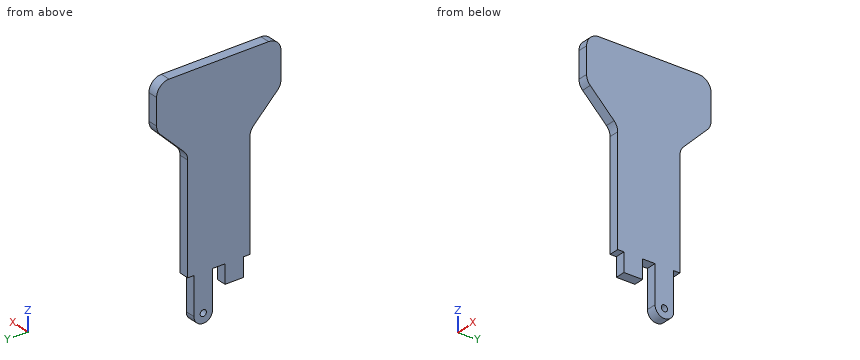
Autodesk Inventor part; units mm, degrees
ref_plane "YZ Plane" through (0, 0, 0) normal (1, 0, 0) x (0, 1, 0)
ref_plane "XZ Plane" through (0, 0, 0) normal (0, 1, 0) x (-1, 0, 0)
ref_plane "XY Plane" through (0, 0, 0) normal (0, 0, 1) x (1, 0, 0)
sketch "Sketch1" plane through (0, 0, 0) normal (1, 0, 0) x (0, 1, 0)
  line L0 (0, 0) -> (1, 0)
  line L1 (1, 0) -> (1, -3)
  line L2 (1, -3) -> (4, -3)
  line L3 (4, -3) -> (4, 0)
  line L4 (4, 0) -> (5, 0)
  line L5 (5, 0) -> (5, 18)
  line L6 (5, 18) -> (10, 23)
  line L7 (10, 23) -> (10, 30)
  line L8 (10, 30) -> (0, 30)
  line L9 (0, 30) -> (0, 0)
  dimension "d0" = 1
  dimension "d1" = 3
  dimension "d2" = 1
  dimension "d3" = 3
  dimension "d4" = 30
  dimension "d5" = 7
  dimension "d6" = 45
  dimension "d7" = 10
extrude "Extrusion1" add sketch "Sketch1" along normal blind 1.6
mirror "Mirror1" about plane through (0, 0, 30) normal (0, -1, 0) of "Extrusion1"
fillet "Fillet1" radius 2 6 edges at (0.8, 10, 30) (0.8, 10, 23) (0.8, -10, 30) (0.8, -10, 23) (0.8, -5, 18) (0.8, 5, 18)
sketch "Sketch2" plane through (1.6, 0, 0) normal (1, 0, 0) x (0, 0, -1)
  line L0 (0, 1) -> (3, 1)
  line L1 (3, 1) -> (3, 4)
  arc A0 (6, 1) -> (6, 4) centre (6, 2.5) ccw
  line L2 (3, 4) -> (6, 4)
  line L3 (3, 1) -> (6, 1)
  circle A1 centre (6, 2.5) radius 0.5
  point P0 (0, 0)
  dimension "d11" = 3
  dimension "d12" = 3
  dimension "d13" = 1
extrude "Extrusion2" add sketch "Sketch2" against normal up to surface (1.6 mm away)
sketch "Sketch3" plane through (1.6, 0, 0) normal (1, 0, 0) x (0, 0, -1)
  line L0 (-30, 10) -> (7.5, 10) construction
  line L1 (7.5, 10) -> (7.5, -9.9928) construction
  line L2 (7.5, -9.9928) -> (-30, -9.9928) construction
  line L3 (-30, -9.9928) -> (-30, 10) construction
  line L4 (-23.8284, 10) -> (-28, 10)
  line L5 (-30, 8) -> (-30, -8)
  arc A0 (6, 1) -> (6, 4) centre (6, 2.5) ccw
  point P0 (0, 0)
  dimension "d17" = 1.5
  dimension "d18" = 1.5
decal "Decal1"
sketch "Sketch4" plane through (0, 0, 0) normal (-1, 0, 0) x (0, 0, 1)
  line L0 (-7.5, 10) -> (30, 10) construction
  line L1 (30, 10) -> (30, -9.9928) construction
  line L2 (30, -9.9928) -> (-7.5, -9.9928) construction
  line L3 (-7.5, -9.9928) -> (-7.5, 10) construction
  line L4 (30, 8) -> (30, -8)
  line L5 (23.8284, 10) -> (28, 10)
  arc A0 (-6, 4) -> (-6, 1) centre (-6, 2.5) ccw
  point P0 (0, 0)
  dimension "d20" = 1.5
decal "Decal2"
equation "\"d17\" = d18"
equation "\"d20\" = d18"
properties part number "KeyerPaddle"
Geometry check sheet. Reference: the model listing, model coordinates, mm. Round coordinates to 2 decimals unless told otherwise and drop trailing zeros. Order: outer loops, then holes, each group sorted by start corner. A loop starts at its lowest first (then second) coordinate and runs counter-clockwise, first axis right, second up. Notation, with made-up numbers: (46.5, 66.5) -> (61.5, 66.5) arc R17 ccw to (61.5, 90.5) -> close; hole circle Ø7 at (6, 24.5). An arc over 180 degrees is marked (long way). Use one line per item in the form item = value.
1. Cross-section at C-C, the plane y = 6. Enter the section's corners in (x, z), plus the area to 3 significant figures.
Working result:
outline = (0, 19) -> (1.6, 19) -> (1.6, 30) -> (0, 30) -> close
area = 17.6 mm^2
2. Go/stop test with flat-tipped pins: pin 1 (0.5 mm diameter, centred on x = 1, z = -2, fed in from +Y); pin 2 (0.8 mm diameter, centred on x = 0.5, z = 12.5, fed in from -Y); pin 3 (0.5 mm diameter, centred on x = 0.5, y = -4.5, fed in from -Z). Record where each tip stops, or that it passes through.
Working result:
pin_1 = 4
pin_2 = -5
pin_3 = 0
3. Cross-section at D-D, the plane z = 12. Enter the section's corners in (x, y), plus the area to 3 significant figures.
Working result:
outline = (0, -5) -> (1.6, -5) -> (1.6, 5) -> (0, 5) -> close
area = 16.0 mm^2
4. Scan lines: line 1 along Y through (x, z) = (1.15, -6); line 2 along Y through (x, z) = (0.4, -2); line 3 along Z through (x, y) = (1.45, -0.5). Record each from-to range of solid material in increasing order. Write a range as from..to.
Working result:
line_1 = 1..2, 3..4
line_2 = -4..-1, 1..4
line_3 = 0..30
5. Cross-section at B-B, the plane x = 0.55. Enter the section's corners in (y, z), plus the area to 3 significant figures.
Working result:
outline = (-10, 23.83) arc R2 ccw to (-9.41, 22.41) -> (-5.59, 18.59) arc R2 cw to (-5, 17.17) -> (-5, 0) -> (-4, 0) -> (-4, -3) -> (-1, -3) -> (-1, 0) -> (1, 0) -> (1, -6) arc R1.5 ccw to (4, -6) -> (4, 0) -> (5, 0) -> (5, 17.17) arc R2 cw to (5.59, 18.59) -> (9.41, 22.41) arc R2 ccw to (10, 23.83) -> (10, 28) arc R2 ccw to (8, 30) -> (-8, 30) arc R2 ccw to (-10, 28) -> close; hole circle Ø1 at (2.5, -6)
area = 423 mm^2
6. Cross-section at A-A, the plane y = 2.5. Enter the section's corners in (x, z), plus the area to 3 significant figures.
Working result:
outline = (0, -7.5) -> (1.6, -7.5) -> (1.6, -6.5) -> (0, -6.5) -> close; (0, -5.5) -> (1.6, -5.5) -> (1.6, 30) -> (0, 30) -> close
area = 58.4 mm^2
